Read the model definition and answer for the solid it produces. Units are mm, in the model's axes. A direction names the side the tool comes from. Round coordinates to 2 decimals unless told otherwise and drop trailing zeros. Order: outer loops, then holes, each group sorted by start corner. A loop starts at its lowest first (then second) coordinate and runs counter-clockwise, first axis right, second up. Notation, with made-up numbers: (72.5, 73) -> (90.5, 73) arc R15 cw to (90.5, 101) -> close; hole circle Ø4 at (54, -9). An arc over 180 degrees is marked (long way). Use a Markdown table: item, result. Add a question column.
1. Consider L1, parallel to Z at x = -25, y = 0.8; L2, parallel to X at y = 1.5, z = 1; L3, parallel to X at y = 3.25, z = 4. Determine where each line is inside the solid, lowest interval first. Write a range as [from, to].
2. Given pin 1 (2.5 mm diameter, centred on x = 14.5, z = 6.5, fed in from +Y); pin 2 (1 mm diameter, centred on x = -32.5, y = 3.5, fed in from -Z); pin 3 (1.5 mm diameter, centred on x = 16.5, y = 4, fed in from +Z), each flat-ended and moving along its own axis, determine where each tip first touches the part or whether it passes through.
3. Section B-B, the plane y = 4 is taken. Give the vertices of the cut face in (x, z).
4. Section D-D, the plane z = 0 is taken. Give the number of separate pieces and of enclosed holes in the cut face, then the cut area to 3 significant figures.
5. The mould has two halves that part along Z. Classify faces 6 (the face through (29.5, 4.7, -0.1)), 7 (the face through (-27.5, 7, -6)), 8 (the face through (-39.965, 6.521, 9.232)): +Z half, -Z half, draft (parallel to the pull), parting line (faces both ways), or undercut.
6. For faces 1 (the face through (15.1, 4.7, 4.5)), 2 (the face through (49, 8, 0)), 3 (the face through (27.5, 1.3, 0.1)), 4 (the face through (0.735, 3.986, -9.232)), 5 (the face through (22.5, 7, 7)), determine the directions among +Z, -Z, +X, -X, +Y, -Y from which every point of the face is accessible in a straight line to the end or side of a thin tool.
7. Section A-A, the plane x = -25 is taken. Give the vertices of the cut face in (y, z), then the cut area to 3 significant figures.
8. Section C-C, the plane x = 8.5 is taken. Give the vertices of the cut face in (y, z).
```python
from build123d import *

# Parameters (mm, degrees)
EXTRUDE_1_DEPTH          = 52.5
SKETCH_2_W               = 5
SKETCH_2_H               = 21
CUT_EXTRUDE_1_DEPTH      = 3
CUT_EXTRUDE_2_DEPTH      = 55.13409277
CUT_EXTRUDE_2_DEPTH_BACK = 55.13409277
SKETCH_3_R               = 2.5
CUT_EXTRUDE_3_DEPTH      = 55.13409277
SKETCH_5_R               = 4.5
CUT_EXTRUDE_4_DEPTH      = 5.5


with BuildPart() as part:
    # 草图1 → 凸台-拉伸1 (new, symmetric)
    with BuildSketch(Plane(origin=(0, 0, 0), x_dir=(0, 0, -1), z_dir=(1, 0, 0))):
        Polygon((-8, 0), (8, 0), (8, 3), (10.5, 5), (8, 8), (-8, 8), (-10.5, 5), (-8, 3), align=None)
    extrude(amount=EXTRUDE_1_DEPTH, both=True)

    # 草图2 → 切除-拉伸1 (cut)
    with BuildSketch(Plane(origin=(0, 8, 0), x_dir=(1, 0, 0), z_dir=(0, 1, 0))):
        with Locations((-5, 0)):
            Rectangle(SKETCH_2_W, SKETCH_2_H)
        with Locations((45, 0)):
            Rectangle(SKETCH_2_W, SKETCH_2_H)
        with Locations((-15, 0)):
            Rectangle(SKETCH_2_W, SKETCH_2_H)
        with Locations((-25, 0)):
            Rectangle(SKETCH_2_W, SKETCH_2_H)
        with Locations((-35, 0)):
            Rectangle(SKETCH_2_W, SKETCH_2_H)
        with Locations((-45, 0)):
            Rectangle(SKETCH_2_W, SKETCH_2_H)
        with Locations((35, 0)):
            Rectangle(SKETCH_2_W, SKETCH_2_H)
        with Locations((25, 0)):
            Rectangle(SKETCH_2_W, SKETCH_2_H)
        with Locations((15, 0)):
            Rectangle(SKETCH_2_W, SKETCH_2_H)
        with Locations((5, 0)):
            Rectangle(SKETCH_2_W, SKETCH_2_H)
    extrude(amount=-CUT_EXTRUDE_1_DEPTH, mode=Mode.SUBTRACT)

    # 草图3 → 切除-拉伸2 (cut, two sides: drawn at the far end of the back side and taken through both)
    with BuildSketch(Plane.XZ.offset(-CUT_EXTRUDE_2_DEPTH_BACK)):
        with Locations(Location((-25, 0, 0), (0, 0, 180))):
            Circle(SKETCH_3_R)
        with BuildLine():
            Line((5, 2.5), (25, 2.5))
            ThreePointArc((25, 2.5), (27.5, 0), (25, -2.5))
            Line((25, -2.5), (5, -2.5))
            ThreePointArc((5, -2.5), (2.5, 0), (5, 2.5))
        make_face()
    extrude(amount=CUT_EXTRUDE_2_DEPTH + CUT_EXTRUDE_2_DEPTH_BACK, mode=Mode.SUBTRACT)

    # 草图4 → 切除-拉伸3 (cut, symmetric)
    with BuildSketch(Plane.XY):
        Polygon((-52.5, 6), (-50.5, 8), (-52.5, 8), align=None)
    cut_extrude_3 = extrude(amount=CUT_EXTRUDE_3_DEPTH, both=True, mode=Mode.SUBTRACT)

    # 镜向1: 切除-拉伸3 across plane
    add(cut_extrude_3.mirror(Plane(origin=(0, 0, 0), x_dir=(0, 0, 1), z_dir=(1, 0, 0))), mode=Mode.SUBTRACT)

    # 草图5 → 切除-拉伸4 (cut)
    # profile 1 of 2: a face of its own
    with BuildSketch(Plane(origin=(0, 8, 0), x_dir=(1, 0, 0), z_dir=(0, 1, 0))):
        with Locations(Location((-25, 0, 0), (0, 0, 270))):
            Circle(SKETCH_5_R)
    # profile 2 of 2: a face of its own
    with BuildSketch(Plane(origin=(0, 8, 0), x_dir=(1, 0, 0), z_dir=(0, 1, 0))):
        with BuildLine():
            Line((5, 4.5), (25, 4.5))
            ThreePointArc((25, 4.5), (29.5, 0), (25, -4.5))
            Line((25, -4.5), (5, -4.5))
            ThreePointArc((5, -4.5), (0.5, 0), (5, 4.5))
        make_face()
        with BuildLine():
            Line((7.5, -2.5), (5, -2.5))
            ThreePointArc((5, -2.5), (3.232233047, -1.767766953), (2.5, 0))
            ThreePointArc((2.5, 0), (3.232233047, 1.767766953), (5, 2.5))
            Line((5, 2.5), (7.5, 2.5))
            Line((7.5, 2.5), (12.5, 2.5))
            Line((12.5, 2.5), (17.5, 2.5))
            Line((17.5, 2.5), (22.5, 2.5))
            Line((22.5, 2.5), (25, 2.5))
            ThreePointArc((25, 2.5), (26.767766953, 1.767766953), (27.5, 0))
            ThreePointArc((27.5, 0), (26.767766953, -1.767766953), (25, -2.5))
            Line((25, -2.5), (22.5, -2.5))
            Line((22.5, -2.5), (17.5, -2.5))
            Line((17.5, -2.5), (12.5, -2.5))
            Line((12.5, -2.5), (7.5, -2.5))
        make_face(mode=Mode.SUBTRACT)
    extrude(amount=-CUT_EXTRUDE_4_DEPTH, mode=Mode.SUBTRACT)


solid = part.part
```
Verdict:
| question | item | result |
|---|---|---|
| 1 | L1 | z = [-8, -2.5], [2.5, 8] |
| 1 | L2 | x = [-52.5, -27.29], [-22.71, 2.71], [27.29, 52.5] |
| 1 | L3 | x = [-52.5, -27.06], [-22.94, 2.94], [27.06, 52.5] |
| 2 | pin 1 | stops at y = 5 |
| 2 | pin 2 | stops at z = -9.25 |
| 2 | pin 3 | stops at z = 10.19 |
| 3 | outline | (-52.5, -9.25) -> (52.5, -9.25) -> (52.5, 9.25) -> (-52.5, 9.25) -> close; hole circle Ø9 at (-25, 0); hole (5, -4.5) -> (25, -4.5) arc R4.5 ccw to (25, 4.5) -> (5, 4.5) arc R4.5 ccw to start |
| 4 | separate pieces | 3 |
| 4 | enclosed holes | 0 |
| 4 | area | 462 mm2 |
| 5 | face 6 | undercut |
| 5 | face 7 | draft |
| 5 | face 8 | +Z half |
| 6 | face 1 | +Y |
| 6 | face 2 | +Z, -Z, +X, -X, +Y |
| 6 | face 3 | +Y, -Y |
| 6 | face 4 | -Z, +X, -X, -Y |
| 6 | face 5 | +Z, -Z, +Y |
| 7 | outline | (0, -8) -> (3, -8) -> (5, -10.5) -> (5, -4.5) -> (2.5, -4.5) -> (2.5, -2.5) -> (0, -2.5) -> close; (0, 2.5) -> (2.5, 2.5) -> (2.5, 4.5) -> (5, 4.5) -> (5, 10.5) -> (3, 8) -> (0, 8) -> close |
| 7 | area | 50.0 mm2 |
| 8 | outline | (0, -8) -> (3, -8) -> (5, -10.5) -> (8, -8) -> (8, -4.5) -> (2.5, -4.5) -> (2.5, -2.5) -> (0, -2.5) -> close; (0, 2.5) -> (2.5, 2.5) -> (2.5, 4.5) -> (8, 4.5) -> (8, 8) -> (5, 10.5) -> (3, 8) -> (0, 8) -> close |
